CAD build for the part. Positions are in the model's coordinates, mm. Face numbers are marked on the shaded views. Coordinates: 2 decimals unless noted, no trailing zeros. Order: outer loops, then holes, each group sorted by start corner. A loop starts at its lowest first (then second) coordinate and runs counter-clockwise, first axis right, second up. Notation, with made-up numbers: M 17,-17.75 L 25,-17.75 A21 ccw 25,-0.75 Z; hole C 74.25,20 d9. An arc over 180 degrees is marked long. Write item = value, one per line.
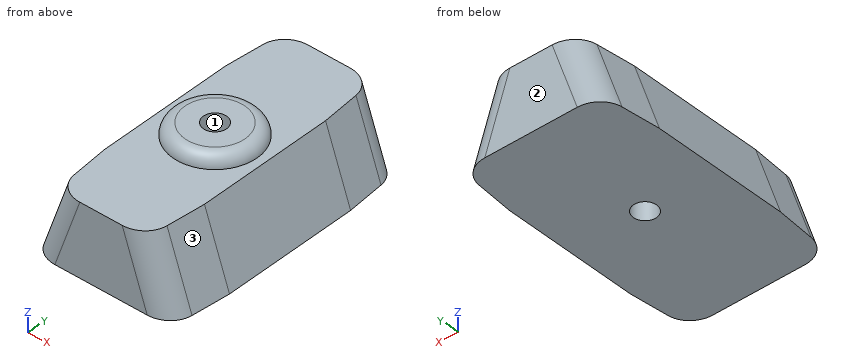
from build123d import *

# Parameters (mm, degrees)
F1_DEPTH   = 16
F2_R       = 5.25
F3_DEPTH   = 1.5
F4_R       = 1.45
F5_DEPTH   = 12
F6_SIZE2   = 0.6561649764
F6_SIZE    = 7.5
F6_2_SIZE2 = 0.6561649764
F6_2_SIZE  = 7.5
F7_R       = 3
F8_R       = 1.49999


# Not quite as in the source:
# - a fillet or chamfer is up to 0.001 mm smaller than in the source, because OpenCascade refuses the exact size


with BuildPart() as f1:
    # F0 (on Front) → F1 (new body, symmetric)
    with BuildSketch(Plane.XZ):
        Polygon((6.25, 0), (0, 0), (-6.25, 0), (-9.375, -9), (0, -9), (9.375, -9), align=None)
    extrude(amount=F1_DEPTH, both=True)

    # F2 (on face) → F3 (join)
    with BuildSketch(Plane.XY):
        Circle(F2_R)
    extrude(amount=F3_DEPTH)

    # F4 (on face) → F5 (cut)
    with BuildSketch(Plane.XY.offset(1.5)):
        Circle(F4_R)
    extrude(amount=-F5_DEPTH, mode=Mode.SUBTRACT)

    # F6
    f6_edges = [f1.edges().sort_by_distance(p)[0] for p in [
        (7.8125, -16, -4.5),
        (7.8125, 16, -4.5),
    ]]
    f6_side = f1.faces().sort_by_distance((7.8125, 0, -4.5))[0]
    chamfer(f6_edges, length=F6_SIZE, length2=F6_SIZE2, reference=f6_side)

    # F6#2
    f6_2_edges = [f1.edges().sort_by_distance(p)[0] for p in [
        (-7.8125, -16, -4.5),
        (-7.8125, 16, -4.5),
    ]]
    f6_2_side = f1.faces().sort_by_distance((-7.8125, 0, -4.5))[0]
    chamfer(f6_2_edges, length=F6_2_SIZE, length2=F6_2_SIZE2, reference=f6_2_side)

    # F7
    f7_edges = [f1.edges().sort_by_distance(p)[0] for p in [
        (7.117906, -16, -4.5),
        (-7.117906, -16, -4.5),
        (7.117906, 16, -4.5),
        (-7.117906, 16, -4.5),
    ]]
    fillet(f7_edges, radius=F7_R)

    # F8 (radius 1.5 in the source; OpenCascade refuses exactly that, so slightly less here)
    f8_edges = [f1.edges().sort_by_distance(p)[0] for p in [
        (-5.25, 0, 1.5),
    ]]
    fillet(f8_edges, radius=F8_R)


solid = f1.part
(1) Slice it at D-D, the plane y = 12. Write the cut outline in (x, z).
Evaluation:
outline = M -9.05,-9 L 9.05,-9 L 5.93,0 L -5.93,0 Z
(2) Slice it at C-C, the plane y = -11. Write the cut outline in (x, z), then the cut area to 3 significant figures.
Evaluation:
outline = M -9.14,-9 L 9.14,-9 L 6.02,0 L -6.02,0 Z
area = 136 mm²
(3) Pin check, flat tips, straight feed: pin 1 Ø4 at (x, y) = (-7, 7) entering from +Z; pin 2 Ø1.5 at (y, z) = (-4, -1) entering from +X; pin 3 Ø1.5 at (y, z) = (-3, -4) entering from +X. Stop position of each tip, or through.
Evaluation:
pin_1 = 0
pin_2 = 6.86
pin_3 = 7.9
(4) Pull direction X, two halves, no side cores. Call the marked faces 1, 2 and 3: +X half, -X half, draft (parallel to the pull), parting line (faces both ways), or undercut.
Evaluation:
face_1 = undercut
face_2 = draft
face_3 = +X half
(5) Wall check: line 1 (Y direction, x = 0, z = -4.5); line 2 (Z direction, x = 4, y = 5); line 3 (Y direction, x = 0.5, z = 0.75). Give the ranges that are in metal, low to high. Write a range as from..to.
Evaluation:
line_1 = -16..-1.45, 1.45..16
line_2 = -9..0
line_3 = -5.02..-1.36, 1.36..5.02
